Read the model definition and answer for the solid it produces. Units are mm, in the model's axes. A direction names the side the tool comes from. Coordinates: 2 decimals unless noted, no trailing zeros. Write each loop counter-clockwise with the first axis right and the second up, starting at its lowest first coordinate (ties: lowest second). Pieces come first, ordered by that corner, then holes. Notation, with made-up numbers: M 46,84.5 L 87,84.5 A16 cw 87,109.5 Z; hole C 85,68.25 d9. An arc over 180 degrees is marked long. Use a Markdown table: item, result. Add a question column.
from build123d import *

# Parameters (mm, degrees)
SKETCH2_W           = 3.35
SKETCH2_H           = 3.35
BOSS_EXTRUDE1_DEPTH = 16.586038969
SKETCH4_R           = 1.8288
CUT_EXTRUDE1_DEPTH  = 27.291440529


with BuildPart() as part:
    # Sketch2 → Boss-Extrude1 (new body)
    with BuildSketch(Plane.XY):
        with BuildLine():
            Line((-0.05, 19.933147112), (-0.05, 12.95))
            Line((-0.05, 12.95), (11.45, 12.95))
            Line((11.45, 12.95), (11.45, 8))
            Line((11.45, 8), (11.45, 3.05))
            Line((11.45, 3.05), (-0.05, 3.05))
            Line((-0.05, 3.05), (-0.05, -3.933147112))
            ThreePointArc((-0.05, -3.933147112), (-8.95, 8), (-0.05, 19.933147112))
        make_face()
        with Locations((0, 8)):
            Rectangle(SKETCH2_W, SKETCH2_H, mode=Mode.SUBTRACT)
    extrude(amount=-BOSS_EXTRUDE1_DEPTH)

    # Sketch4 → Cut-Extrude1 (cut, through all)
    with BuildSketch(Plane.XZ.offset(-3.05)):
        with Locations((6.35, -9)):
            Circle(SKETCH4_R)
    extrude(amount=-CUT_EXTRUDE1_DEPTH, mode=Mode.SUBTRACT)


solid = part.part
Item 1: Find section A-A on x = 6.35. Give the vertices of the cut face in (y, z).
Item 2: Each of these flat-tipped pins is pushed along its axis until it touches: pin 1 (7.5 mm diameter, centred on y = 17.5, z = -4.5, fed in from +X); pin 2 (3.5 mm diameter, centred on x = 0, z = -11.5, fed in from -Y); pin 3 (9 mm diameter, centred on x = 5, z = -9, fed in from -Y). Where does it stop, or does it pass through?
Item 3: Consider probe 1 along Z at (x, y) = (6.35, 6.25); probe 2 along X at (y, z) = (8, -15) (3 decimals); probe 3 along X at (y, z) = (7.75, -8.75) (3 decimals). Determine where each line is inside the solid, lowest interval first.
Item 4: Find section D-D on y = 10.75. Give the vertices of the cut face in (x, z).
Item 5: Find section B-B on z = -9. Give the vertices of the cut face in (x, y) (3 decimals).
Item 6: For faces 5 (the flat face through (1.675, 8, -8)), 6 (the flat face through (4, 12.95, -8)), 7 (the flat face through (-1, 6, 0)), determine the directions among +Z, -Z, +X, -X, +Y, -Y from which every point of the face is accessible in a straight line to the end or side of a thin tool.
Item 7: Determine the mould class of faces 1 (the flat face through (0, 6.325, -8)), 2 (the flat face through (4.5, 3.05, -8.2)), 3 (the flat face through (-0.05, 0, -8)), 4 (the cylindrical face through (-8.95, 7.78, -8.18)) for opening direction Y: pulls with the +Y half, pulls with the -Y half, needs draft (parallel to the pull), parting line crosses it, or undercut.
Item 8: Find section C-C on z = -11.75. Give the vertices of the cut face in (x, y) (3 decimals), then the cut area to 3 significant figures.
Geometry says:
| question | item | result |
|---|---|---|
| 1 | outline | M 3.05,-16.59 L 12.95,-16.59 L 12.95,-10.83 L 3.05,-10.83 Z; M 3.05,-7.17 L 12.95,-7.17 L 12.95,0 L 3.05,0 Z |
| 2 | pin 1 | stops at x = -0.05 |
| 2 | pin 2 | stops at y = -3.93 |
| 2 | pin 3 | stops at y = 3.05 |
| 3 | probe 1 | z = -16.59 to -10.83, -7.17 to 0 |
| 3 | probe 2 | x = -8.95 to -1.675, 1.675 to 11.45 |
| 3 | probe 3 | x = -8.947 to -1.675, 1.675 to 4.538, 8.162 to 11.45 |
| 4 | outline | M -8.64,-16.59 L 11.45,-16.59 L 11.45,0 L -8.64,0 Z; hole C 6.35,-9 d3.66 |
| 5 | outline | M -0.05,-3.933 L -0.05,3.05 L 4.521,3.05 L 4.521,12.95 L -0.05,12.95 L -0.05,19.933 A12.45 ccw Z; M 8.179,3.05 L 11.45,3.05 L 11.45,12.95 L 8.179,12.95 Z; hole M -1.675,6.325 L 1.675,6.325 L 1.675,9.675 L -1.675,9.675 Z |
| 6 | face 5 | +Z, -Z |
| 6 | face 6 | +Z, -Z, +X, +Y |
| 6 | face 7 | +Z, +X, -X, +Y, -Y |
| 7 | face 1 | undercut |
| 7 | face 2 | pulls with the -Y half |
| 7 | face 3 | needs draft |
| 7 | face 4 | parting line crosses it |
| 8 | outline | M -0.05,-3.933 L -0.05,3.05 L 11.45,3.05 L 11.45,12.95 L -0.05,12.95 L -0.05,19.933 A12.45 ccw Z; hole M -1.675,6.325 L 1.675,6.325 L 1.675,9.675 L -1.675,9.675 Z |
| 8 | area | 259 mm2 |
